Autodesk Inventor part; units mm, degrees
ref_plane "YZ Plane" through (0, 0, 0) normal (1, 0, 0) x (0, 1, 0)
ref_plane "XZ Plane" through (0, 0, 0) normal (0, 1, 0) x (-1, 0, 0)
ref_plane "XY Plane" through (0, 0, 0) normal (0, 0, 1) x (1, 0, 0)
sketch "Skizze1" plane through (0, 0, 0) normal (0, 0, 1) x (1, 0, 0)
  line L0 (-80, 25) -> (80, 25)
  line L1 (80, 25) -> (80, -50)
  line L2 (80, -50) -> (-80, -50)
  line L3 (-80, -50) -> (-80, 25)
  line L4 (-112, 0) -> (112, 0)
  line L5 (0, -65) -> (0, 40)
  circle A0 centre (-30, 0) radius 2.7
  circle A1 centre (30, 0) radius 2.7
  point P0 (0, 0)
  dimension "d0" = 25
  dimension "d1" = 160
  dimension "d2" = 60
  dimension "d3" = 5.4
  dimension "d4" = 75
extrude "Extrusion1" add sketch "Skizze1" along normal blind 10 contours L0 L5 L4 A0 L3 | L0 L1 L4 A1 L5 | L4 A0 L5 L2 L3 | L4 A1 L1 L2 L5
sketch "Skizze3" plane through (0, 0, 10) normal (0, 0, 1) x (1, 0, 0)
  circle A0 centre (30, 0) radius 2.7
  circle A1 centre (-30, 0) radius 2.7
  circle A2 centre (-30, 0) radius 7
  circle A3 centre (30, 0) radius 7
  point P0 (0, 0)
  dimension "d8" = 14
extrude "Extrusion2" cut sketch "Skizze3" against normal blind 6
sketch "Skizze4" plane through (0, 0, 0) normal (0, 0, -1) x (-1, 0, 0)
  line L0 (80, 25) -> (-80, 25)
  line L1 (-80, 25) -> (-80, -50)
  line L2 (-80, -50) -> (80, -50)
  line L3 (80, -50) -> (80, 25)
  line L4 (0, -50) -> (0, 25)
  line L5 (-65, -50) -> (-65, 25)
  line L6 (65, -50) -> (65, 25)
  line L7 (-80, -12.5) -> (80, -12.5)
  point P0 (0, 0)
  point P1 (-65, 7.5)
  point P2 (-65, -32.5)
  point P3 (65, -32.5)
  point P4 (65, 7.5)
  dimension "d11" = 130
  dimension "d12" = 40
hole "Bohrung1" at (65, 7.5, 0) at (65, -32.5, 0) at (-65, -32.5, 0) at (-65, 7.5, 0) direction (0, 0, 1) diameter 4.5 end through all counterbore diameter 8 counterbore depth 6
properties part number "1_0204_012"
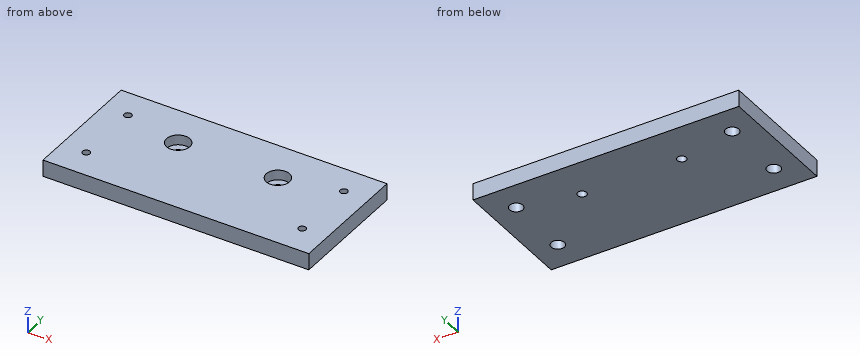
Could you check a few things on this model? Use its own coordinates, in mm. Give positions to 0.01 mm unless a question says otherwise; leave off trailing zeros. Write each loop counter-clockwise with the first axis right and the second up, starting at its lowest first coordinate (ties: lowest second). Pieces come first, ordered by that corner, then holes. Notation, with made-up numbers: (-1.5, 83) -> (45.5, 83) arc R12 cw to (45.5, 96) -> close; hole circle Ø9 at (6.5, 5). An arc over 180 degrees is marked (long way). Answer as a JSON object with one key per item and string values.
Q1. Suppose I cut it at A-A on x = -65. Write out the boundary of the cut face in (y, z), then the cut area to 3 significant figures.
Taken from the geometry:
{"outline": "(-50, 0) -> (-36.5, 0) -> (-36.5, 6) -> (-34.75, 6) -> (-34.75, 10) -> (-50, 10) -> close; (-30.25, 6) -> (-28.5, 6) -> (-28.5, 0) -> (3.5, 0) -> (3.5, 6) -> (5.25, 6) -> (5.25, 10) -> (-30.25, 10) -> close; (9.75, 6) -> (11.5, 6) -> (11.5, 0) -> (25, 0) -> (25, 10) -> (9.75, 10) -> close", "area": "618 mm²"}
Q2. Suppose I cut it at C-C on z = 2.25. Write out the boundary of the cut face in (x, y).
Taken from the geometry:
{"outline": "(-80, -50) -> (80, -50) -> (80, 25) -> (-80, 25) -> close; hole circle Ø8 at (-65, -32.5); hole circle Ø8 at (-65, 7.5); hole circle Ø5.4 at (-30, 0); hole circle Ø5.4 at (30, 0); hole circle Ø8 at (65, -32.5); hole circle Ø8 at (65, 7.5)"}
Q3. Please list where these lines run through material, in increasing order: L1, parallel to X at y = -32.5, z = 2.95; L2, parallel to X at y = -32.5, z = 7.55; L3, parallel to Y at x = -65, z = 5.
Taken from the geometry:
{"L1": "x = -80 to -69, -61 to 61, 69 to 80", "L2": "x = -80 to -67.25, -62.75 to 62.75, 67.25 to 80", "L3": "y = -50 to -36.5, -28.5 to 3.5, 11.5 to 25"}
Q4. Will these pins go through, and if not, where does the flat tip stop? pin 1 Ø7 at (x, y) = (-65, 7.5) entering from +Z; pin 2 Ø5 at (x, y) = (65, 7.5) entering from -Z; pin 3 Ø8.5 at (x, y) = (30, 0) entering from +Z; pin 4 Ø2.5 at (x, y) = (-65, -32.5) entering from -Z.
Taken from the geometry:
{"pin 1": "stops at z = 10", "pin 2": "stops at z = 6", "pin 3": "stops at z = 4", "pin 4": "passes through"}
Q5. Suppose I cut it at D-D on x = -30. Write out the boundary of the cut face in (y, z), then the cut area to 3 significant figures.
Taken from the geometry:
{"outline": "(-50, 0) -> (-2.7, 0) -> (-2.7, 4) -> (-7, 4) -> (-7, 10) -> (-50, 10) -> close; (2.7, 0) -> (25, 0) -> (25, 10) -> (7, 10) -> (7, 4) -> (2.7, 4) -> close", "area": "644 mm²"}
Q6. Suppose I cut it at B-B on y = -32.5. Write out the boundary of the cut face in (x, z).
Taken from the geometry:
{"outline": "(-80, 0) -> (-69, 0) -> (-69, 6) -> (-67.25, 6) -> (-67.25, 10) -> (-80, 10) -> close; (-62.75, 6) -> (-61, 6) -> (-61, 0) -> (61, 0) -> (61, 6) -> (62.75, 6) -> (62.75, 10) -> (-62.75, 10) -> close; (67.25, 6) -> (69, 6) -> (69, 0) -> (80, 0) -> (80, 10) -> (67.25, 10) -> close"}
